Print and shaded views of the part. All mm, measured from the part's lowest x, y and z. A direction names the side the tool comes from. Give positions to 0.01 mm unless a question says otherwise; leave off trailing zeros. Loops run counter-clockwise (first coordinate to the right, second up) from the corner with the lowest first, then second, coordinate; pieces in that order, holes last. Notation, with made-up numbers: M -29,12 L -12,12 A16 ccw -12,38 Z; hole C 69.5,24.25 d2. An arc over 180 degrees is marked long. Answer as CSV lines item,"result".
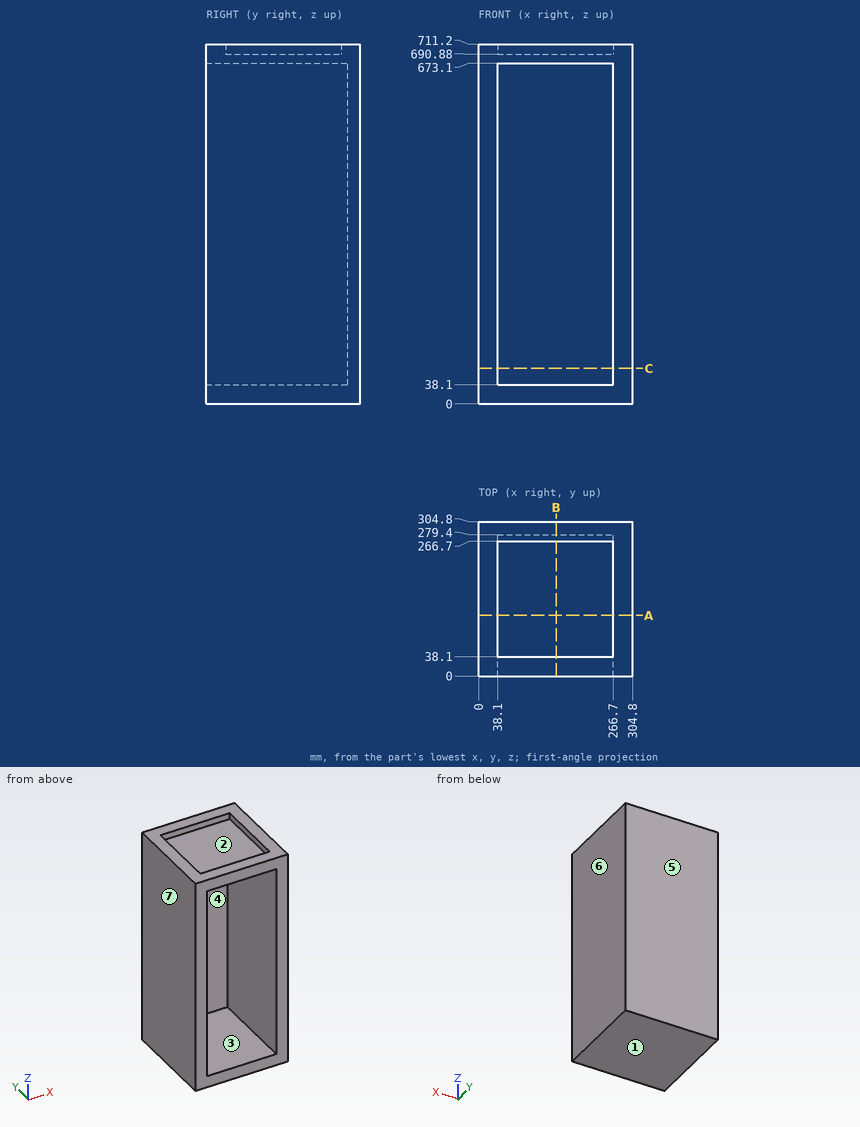
Q1. Cut at B-B (x = 153.5). Write the cut outline in (y, z), and give its area (3 significant figures).
Solution:
outline,"M 0,0 L 304.8,0 L 304.8,711.2 L 266.7,711.2 L 266.7,690.88 L 38.1,690.88 L 38.1,711.2 L 0,711.2 L 0,673.1 L 279.4,673.1 L 279.4,38.1 L 0,38.1 Z"
area,"34,700 mm²"
Q2. Which spindle directions (+Z, -Z, +X, -X, +Y, -Y) get a long thin tool onto all of the face, cutting with end or side? Do the marked faces 1, 2 and 3. Say none if no direction does.
Solution:
face 1,"-Z, +X, -X, +Y, -Y"
face 2,"+Z"
face 3,"-Y"
Q3. Pin check, flat tips, straight feed: P1, Ø22.5, axis at x = 101.5, z = 704.5, coming from the -Y side; P2, Ø4, axis at x = 97, y = 145, coming from the +Z side; P3, Ø4, axis at x = 172, z = 483, coming from the -Y side. Stop position of each tip, or through.
Solution:
P1,"stops at y = 0"
P2,"stops at z = 690.88"
P3,"stops at y = 279.4"
Q4. Wall check: line 1 (X direction, y = 203, z = 483); line 2 (Z direction, x = 163, y = 227.5); line 3 (Z direction, x = 83, y = 27). Give the ranges that are in metal, low to high. Write a range as [from, to].
Solution:
line 1,"x = [0, 38.1], [266.7, 304.8]"
line 2,"z = [0, 38.1], [673.1, 690.88]"
line 3,"z = [0, 38.1], [673.1, 711.2]"
Q5. Cut at A-A (y = 120). Write the cut outline in (x, z), and give its area (3 significant figures).
Solution:
outline,"M 0,0 L 304.8,0 L 304.8,711.2 L 266.7,711.2 L 266.7,690.88 L 38.1,690.88 L 38.1,711.2 L 0,711.2 Z; hole M 38.1,38.1 L 266.7,38.1 L 266.7,673.1 L 38.1,673.1 Z"
area,"67,000 mm²"
Q6. Cut at C-C (z = 70). Write the cut outline in (x, y).
Solution:
outline,"M 0,0 L 38.1,0 L 38.1,279.4 L 266.7,279.4 L 266.7,0 L 304.8,0 L 304.8,304.8 L 0,304.8 Z"
Q7. Mould opens along X. For the marked faces 4, 5, 6 and 7 say: released by +X, released by -X, zero draft, split by the parting line, or undercut.
Solution:
face 4,"undercut"
face 5,"zero draft"
face 6,"released by +X"
face 7,"released by -X"
